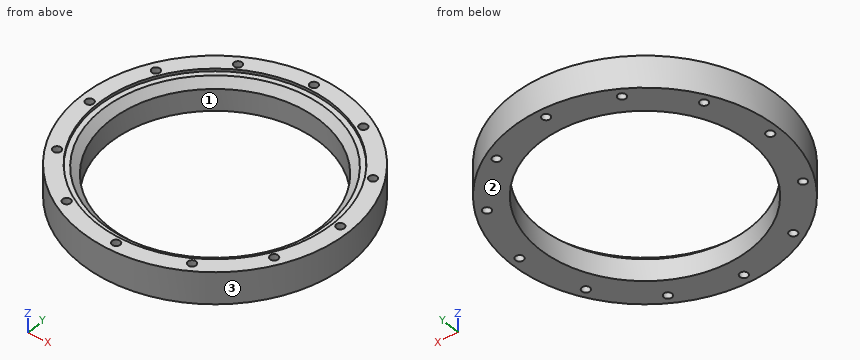
```python
from build123d import *

# Parameters (mm, degrees)
SKETCH_R           = 1.5
POCKET_DEPTH       = 295.86012
POLARPATTERN_COUNT = 12


with BuildPart() as part:
    # Sketch013 → Revolution (revolve)
    with BuildSketch(Plane.XZ):
        Polygon((39.3, 0), (39.3, 8.198781), (42.101219, 11), (44, 11), (44, 12), (50, 12), (50, 0), align=None)
    revolve(axis=Axis((0, 0, 0), (0, 0, 1)))

    # Sketch → Pocket (cut, through all)
    with BuildSketch(Plane(origin=(0, 0, 0), x_dir=(1, 0, 0), z_dir=(0, 0, -1))):
        with Locations((46.4, 0)):
            Circle(SKETCH_R)
    pocket = extrude(amount=-POCKET_DEPTH, mode=Mode.SUBTRACT)

    # PolarPattern: Pocket ×12 about axis
    polarpattern_axis = Axis((0, 0, 0), (0, 0, -1))
    for i in range(1, POLARPATTERN_COUNT):
        add(pocket.rotate(polarpattern_axis, i * 360 / POLARPATTERN_COUNT), mode=Mode.SUBTRACT)


solid = part.part
```
Design review of the part built by this model. Coordinates are the model's own, in mm. Face numbers are marked on the shaded views. Give positions to 0.01 mm unless a question says otherwise; leave off trailing zeros. Loops run counter-clockwise (first coordinate to the right, second up) from the corner with the lowest first, then second, coordinate; pieces in that order, holes last. Notation, with made-up numbers: M 2,26.5 L 11,26.5 A14 ccw 11,44.5 Z; hole C 69,17 d5. An arc over 180 degrees is marked long. Return JSON: item names as keys, results as strings. Group by question number.
Item 1: We need section C-C (x = 46.4). Give the boundary of the cut face in (y, z).
Item 2: For probe 1 along Y at (x, z) = (23.2, 4.5); probe 2 along X at (y, z) = (0.5, 8); probe 3 along Y at (x, z) = (-20, 3.75), list the stretches that pass through material, from the lowest coordinate up.
Item 3: Insertion check: pin 1 Ø1 at (y, z) = (-18.5, 9) entering from -X; pin 2 Ø2 at (x, z) = (3, 5) entering from -Y; pin 3 Ø3 at (x, z) = (33, 5.5) entering from +Y. Each pin has a flat end and moves straight along its axis. Give the tip position at first contact, or say it passes through.
Item 4: Mouldability with a two-part tool opening along Y and no side actions: class the marked faces 1, 2 and 3 as released by +Y, released by -Y, zero draft, split by the parting line, or undercut.
Item 5: We need section A-A (y = 0). Give the boundary of the cut face in (x, z), and give its area (3 significant figures).
Output:
{
 "1": {"outline": "M -18.63,0 L -1.5,0 L -1.5,12 L -18.63,12 Z; M 1.5,0 L 18.63,0 L 18.63,12 L 1.5,12 Z"},
 "2": {"probe 1": "y = -44.29 to -41.68, -38.68 to -31.72, 31.72 to 38.68, 41.68 to 44.29", "probe 2": "x = -50 to -47.81, -44.99 to -39.3, 39.3 to 44.99, 47.81 to 50", "probe 3": "y = -45.83 to -33.83, 33.83 to 45.83"},
 "3": {"pin 1": "stops at x = -46.65", "pin 2": "stops at y = -49.96", "pin 3": "stops at y = 38.83"},
 "4": {"face 1": "undercut", "face 2": "zero draft", "face 3": "split by the parting line"},
 "5": {"outline": "M -50,0 L -47.9,0 L -47.9,12 L -50,12 Z; M -44.9,0 L -39.3,0 L -39.3,8.2 L -42.1,11 L -44,11 L -44,12 L -44.9,12 Z; M 39.3,0 L 44.9,0 L 44.9,12 L 44,12 L 44,11 L 42.1,11 L 39.3,8.2 Z; M 47.9,0 L 50,0 L 50,12 L 47.9,12 Z", "area": "168 mm^2"}
}
